Autodesk Inventor part; units mm, degrees
ref_plane "YZ Plane" through (0, 0, 0) normal (1, 0, 0) x (0, 1, 0)
ref_plane "XZ Plane" through (0, 0, 0) normal (0, 1, 0) x (-1, 0, 0)
ref_plane "XY Plane" through (0, 0, 0) normal (0, 0, 1) x (1, 0, 0)
sketch "Sketch1" plane through (0, 0, 0) normal (0, 0, 1) x (1, 0, 0)
  line L0 (0, 0) -> (-20, 0)
  line L1 (-20, 0) -> (-20, 2)
  line L2 (-20, 2) -> (0, 2)
  line L3 (0, 2) -> (0, 0)
  line L4 (0, 2) -> (2, 2)
  circle A0 centre (2, 2) radius 2
  line L5 (2, 0) -> (0, 0)
  dimension "d0" = 20
  dimension "d1" = 2
  dimension "d2" = 2
extrude "Extrusion1" add sketch "Sketch1" along normal blind 58
sketch "Sketch2" plane through (-20, 2, 0) normal (0, 1, 0) x (1, 0, 0)
  line L0 (22, 0) -> (20, 0)
  line L1 (20, 0) -> (20, -58)
  line L2 (22, -58) -> (20, -58)
  line L3 (22, 0) -> (22, -58)
  line L4 (20, 0) -> (0, 0)
  line L5 (0, 0) -> (0, -58)
  line L6 (20, -58) -> (0, -58)
  line L7 (20, 0) -> (20, -58)
  line L8 (20, 0) -> (24, 0)
  line L9 (24, 0) -> (20, 0)
  line L10 (20, 0) -> (20, -11.6)
  line L11 (20, -11.6) -> (24, -11.6)
  line L12 (24, -11.6) -> (24, 0)
  line L13 (20, -11.6) -> (24, -11.6)
  line L14 (24, -11.6) -> (24, -23.2)
  line L15 (24, -23.2) -> (20, -23.2)
  line L16 (20, -23.2) -> (20, -11.6)
  line L17 (24, -23.2) -> (20, -23.2)
  line L18 (20, -23.2) -> (20, -34.8)
  line L19 (20, -34.8) -> (24, -34.8)
  line L20 (24, -34.8) -> (24, -23.2)
  line L21 (24, 0) -> (24, -58)
  line L22 (20, -34.8) -> (24, -34.8)
  line L23 (24, -34.8) -> (24, -46.4)
  line L24 (24, -46.4) -> (20, -46.4)
  line L25 (20, -46.4) -> (20, -34.8)
  line L26 (24, -46.4) -> (20, -46.4)
  line L27 (20, -46.4) -> (20, -58)
  line L28 (20, -58) -> (24, -58)
  line L29 (24, -58) -> (24, -46.4)
  dimension "d5" = 11.6
  dimension "d6" = 11.6
  dimension "d7" = 11.6
  dimension "d8" = 11.6
extrude "Extrusion2" cut sketch "Sketch2" along normal mid plane 4 contours L3 L11 L1 L0 | L8 L12 L11 L3 | L15 L20 L19 L3 | L3 L19 L1 L15 | L1 L24 L3 L2 | L24 L21 L28 L3
sketch "Sketch3" plane through (0, 0, 58) normal (0, 0, 1) x (1, 0, 0)
  arc A0 (2, 0) -> (0, 2) centre (2, 2) ccw
  line L0 (0, 2) -> (0, 0)
  line L1 (2, 0) -> (0, 0)
hole "Hole1" at (2, 2, 58) direction (0, 0, -1) diameter 3 end through all
properties part number "SchanierTeilB_CPY"
Geometry: final body of the model. Coordinates: model frame, mm. A direction names the side the tool comes from. Give positions to 0.01 mm unless a question says otherwise; leave off trailing zeros. Loops run counter-clockwise (first coordinate to the right, second up) from the corner with the lowest first, then second, coordinate; pieces in that order, holes last. Notation, with made-up numbers: M 2.5,50 L 25.5,50 A26 ccw 25.5,87 Z; hole C 58,12.25 d11. An arc over 180 degrees is marked long. Put each result on its own line as item: value.
1) Mould query, pull axis Z, two halves, no side actions, for faces 5 (the flat face through (0, 1, 29)), 6 (the flat face through (-10, 1, 0)), 7 (the cylindrical face through (3.367, 3.46, 40.519)), 8 (the flat face through (1.1, 0.6, 34.8)). Classes: released by +Z, released by -Z, zero draft, split by the parting line, or undercut.
Computed values:
face 5: undercut
face 6: released by -Z
face 7: zero draft
face 8: undercut
2) Material intervals for L1, parallel to Y at x = 2, z = 18.5; L2, parallel to X at y = 1.85, z = 21; L3, parallel to Y at x = -6.25, z = 2, sorted ascending. Write a range as from..to.
Computed values:
L1: y = 0..0.5, 3.5..4
L2: x = -20..0.51, 3.49..3.99
L3: y = 0..2
3) Cut plane A-A, the plane y = 2.6. Return the cut outline in (x, z), plus the area to 3 significant figures.
Computed values:
outline: M 0.09,11.6 L 0.63,11.6 L 0.63,23.2 L 0.09,23.2 Z; M 0.09,34.8 L 0.63,34.8 L 0.63,46.4 L 0.09,46.4 Z; M 3.37,11.6 L 3.91,11.6 L 3.91,23.2 L 3.37,23.2 Z; M 3.37,34.8 L 3.91,34.8 L 3.91,46.4 L 3.37,46.4 Z
area: 24.7 mm^2
4) Cut plane B-B, the plane z = 26.5. Return the cut outline in (x, y).
Computed values:
outline: M -20,0 L 0,0 L 0,2 L -20,2 Z
5) Reachability of faces 1 (the flat face through (1.1, 0.6, 23.2)), 2 (the flat face through (0, 1, 6)), 3 (the flat face through (1.1, 0.6, 46.4)), 4 (the flat face through (-10, 2, 29)) from +Z, -Z, +X, -X, +Y, -Y: full face, straight path, thin tool, end or side. Return the list, or none.
Computed values:
face 1: +X, +Y, -Y
face 2: -Z, +X, +Y, -Y
face 3: +Z, +X, +Y, -Y
face 4: +Z, -Z, -X, +Y
6) Cut plane C-C, the plane x = -8.25. Return the cut outline in (y, z), plus the area to 3 significant figures.
Computed values:
outline: M 0,0 L 2,0 L 2,58 L 0,58 Z
area: 116 mm^2
7) First-contact query: P1, Ø1.2, axis at x = 2.5, y = 1, coming from the +Z side; P2, Ø6, axis at x = -8.5, z = 26.5, coming from the +Y side; P3, Ø0.6, axis at y = 1, z = 31.5, coming from the +X side. Flat tips, straight axial feed; report the tip coordinate or a pass-through.
Computed values:
P1: stops at z = 46.4
P2: stops at y = 2
P3: stops at x = 0
